Verification items for the finished model (mm, model axes). A direction names the side the tool comes from. Coordinates: 2 decimals unless noted, no trailing zeros. Order: outer loops, then holes, each group sorted by start corner. A loop starts at its lowest first (then second) coordinate and runs counter-clockwise, first axis right, second up. Notation, with made-up numbers: (41.5, 64.5) - (49.5, 64.5) arc R13 cw to (49.5, 82.5) - close; hole circle Ø11 at (56.25, 83.5). An arc over 180 degrees is marked (long way). Answer as CSV lines item,"result". Start each with the question number.
1. Set-up check for faces 1 (the flat face through (0, 6, 28)), 2 (the flat face through (0, -6, 28)), 3 (the flat face through (33, 0, 6)): record each of +Z, -Z, +X, -X, +Y, -Y from which the full face is reachable in a straight line by a thin tool's end or side.
2. Go/stop test with flat-tipped pins: pin 1 (1 mm diameter, centred on y = 3, z = 33, fed in from +X); pin 2 (1.5 mm diameter, centred on x = -13.5, z = 27.5, fed in from +Y); pin 3 (21 mm diameter, centred on x = 0.5, y = -7.5, fed in from +Z). Record where each tip stops, or that it passes through.
3. Material ranges on L1, parallel to X at y = -3, z = 8; L2, parallel to X at y = -8, z = 42; L3, parallel to Y at x = -11.5, z = 30, recorded low to high. Write a range as [from, to].
4. Section check D-D (y = -4.5). Record the cut outline in (x, z).
5. Section check C-C (z = 7.5). Record the cut outline in (x, y).
6. Section check A-A (z = 16). Record the cut outline in (x, y), and give its area (3 significant figures).
Autodesk Fusion 360 part; units mm, degrees
sketch "Sketch1" plane through (0, 0, 0) normal (0, 0, 1) x (1, 0, 0)
  line L0 (33, 21) -> (-33, 21)
  line L1 (-33, 21) -> (-33, -21)
  line L2 (-33, -21) -> (33, -21)
  line L3 (33, -21) -> (33, 21)
  line L4 (33, 21) -> (-33, -21) construction
  line L5 (-33, 21) -> (33, -21) construction
  dimension "d1" = 66
  dimension "d2" = 42
extrude "Extrude1" add sketch "Sketch1" along normal blind 12
chamfer "Chamfer1" distance 12 angle 45 2 edges at (33, -21, 6) (33, 21, 6)
sketch "Sketch2" plane through (0, 0, 12) normal (0, 0, 1) x (-1, 0, 0)
  line L0 (-33, -9) -> (-21, -21)
  line L1 (-21, -21) -> (33, -21)
  line L2 (33, -21) -> (33, 21)
  line L3 (33, 21) -> (-21, 21)
  line L4 (-21, 21) -> (-33, 9)
  line L5 (-33, 9) -> (-33, -9)
  line L6 (33, -21) -> (21, -21)
  line L7 (21, -21) -> (21, 21)
  line L8 (21, 21) -> (33, 21)
  line L9 (33, 21) -> (33, -21)
  dimension "d6" = 12
extrude "Extrude2" add sketch "Sketch2" along normal blind 48 contours L1 L2 L3 L6 L7 L8 L9
fillet "Fillet1" radius 21 2 edges at (-27, -21, 60) (-27, 21, 60)
sketch "Sketch3" plane through (0, 0, 0) normal (0, 1, 0) x (1, 0, 0)
  line L0 (-20.9271, -11.9611) -> (-20.9271, -53.9611)
  line L1 (-20.9271, -11.9611) -> (33.0729, -11.9611)
  line L2 (33.0729, -11.9611) -> (-20.9271, -53.9611)
  dimension "d11" = 42
  dimension "d12" = 54
extrude "Extrude3" add sketch "Sketch3" along normal mid plane 12
equation "d7 = 60 mm - 12 mm"
equation "d12 = 66 mm - 12 mm"
Evaluation:
1,face 1,"+Z, +X, +Y"
1,face 2,"+Z, +X, -Y"
1,face 3,"-Z, +X, +Y, -Y"
2,pin 1,"stops at x = 6.67"
2,pin 2,"stops at y = 6"
2,pin 3,"stops at z = 45.38"
3,L1,"x = [-33, 33]"
3,L2,"x = [-33, -21]"
3,L3,"y = [-6, 6]"
4,outline,"(-33, 0) - (33, 0) - (33, 11.96) - (33.07, 11.96) - (-20.93, 53.96) - (-20.93, 12) - (-21, 12) - (-21, 59.51) - (-33, 59.51) - close"
5,outline,"(-33, -21) - (21, -21) - (33, -9) - (33, 9) - (21, 21) - (-33, 21) - close"
6,outline,"(-33, -21) - (-21, -21) - (-21, 21) - (-33, 21) - close; (-20.93, -6) - (27.88, -6) - (27.88, 6) - (-20.93, 6) - close"
6,area,"1,090 mm²"
